Verification items for the finished model (mm, model axes). A direction names the side the tool comes from. Round coordinates to 2 decimals unless told otherwise and drop trailing zeros. Write each loop counter-clockwise with the first axis right and the second up, starting at its lowest first coordinate (ties: lowest second). Pieces come first, ordered by that corner, then holes. Notation, with made-up numbers: (44.5, 43) - (83.5, 43) arc R19 cw to (83.5, 57) - close; hole circle Ø7 at (64, 80). An arc over 180 degrees is marked (long way). Answer as a JSON object with one key per item and string values.
```python
from build123d import *

# Parameters (mm, degrees)
SKETCH_1_W              = 150
SKETCH_1_H              = 80
EXTRUDE_1_DEPTH         = 2
HOLE_WIZARD_3_2_3_2_1_D = 3.2
FILLET_1_R              = 5
SKETCH_4_W              = 25
SKETCH_4_H              = 60
CUT_EXTRUDE_1_DEPTH     = 86.023526156
FILLET_2_R              = 2


with BuildPart() as part:
    # 草图1 → 凸台-拉伸1 (new body)
    with BuildSketch(Plane(origin=(0, 0, 0), x_dir=(1, 0, 0), z_dir=(0, 1, 0))):
        Rectangle(SKETCH_1_W, SKETCH_1_H)
    extrude(amount=EXTRUDE_1_DEPTH)

    # Ø3.2 (3.2) 直径孔1 (through all)
    with Locations(Plane(origin=(-31, 2, -25), x_dir=(0, 0, 1), z_dir=(0, 1, 0))):
        with Locations((0, 0), (50, 0), (50, 62), (0, 62), (5, -39), (45, -39), (45, 101), (5, 101)):
            Hole(HOLE_WIZARD_3_2_3_2_1_D / 2)

    # 圆角1
    fillet_1_edges = [part.edges().sort_by_distance(p)[0] for p in [
        (75, 1, 40),
        (-75, 1, 40),
        (-75, 1, -40),
        (75, 1, -40),
    ]]
    fillet(fillet_1_edges, radius=FILLET_1_R)

    # 草图4 → 切除-拉伸1 (cut, through all)
    with BuildSketch(Plane(origin=(0, 2, 0), x_dir=(1, 0, 0), z_dir=(0, 1, 0))):
        with Locations((-47.5, 0)):
            Rectangle(SKETCH_4_W, SKETCH_4_H)
        Polygon((-27, 30), (-27, -20), (27, 30), align=None)
        Polygon((-23.081304406, -30), (27, -30), (27, 16.371578153), align=None)
        with Locations((47.5, 0)):
            Rectangle(SKETCH_4_W, SKETCH_4_H)
    extrude(amount=-CUT_EXTRUDE_1_DEPTH, mode=Mode.SUBTRACT)

    # 圆角2
    fillet_2_edges = [part.edges().sort_by_distance(p)[0] for p in [
        (-60, 1, 30),
        (-60, 1, -30),
        (-35, 1, -30),
        (-35, 1, 30),
        (-23.081304406, 1, 30),
        (27, 1, -16.371578153),
        (27, 1, 30),
        (-27, 1, -30),
        (27, 1, -30),
        (-27, 1, 20),
        (60, 1, -30),
        (60, 1, 30),
        (35, 1, 30),
        (35, 1, -30),
    ]]
    fillet(fillet_2_edges, radius=FILLET_2_R)


solid = part.part
```
Q1. Release check for a two-part mould opening along Z. For faces 1 (the flat face through (-1, 0, -1)), 2 (the cylindrical face through (73, 1, 39)), 3 (the cylindrical face through (-31.97, 0.99, 26.27)), 4 (the cylindrical face through (-74, 1, -38)) record: released by +Z, released by -Z, zero draft, split by the parting line, or undercut.
Geometry check:
{"face 1": "zero draft", "face 2": "released by +Z", "face 3": "undercut", "face 4": "released by -Z"}
Q2. Material ranges on line 1 along Z through (x, y) = (70, 1.6); line 2 along X through (y, z) = (1.65, -27); line 3 along Z through (x, y) = (46.5, 0.6), recorded low to high. Write a range as [from, to].
Geometry check:
{"line 1": "z = [-40, -21.6], [-18.4, 18.4], [21.6, 40]", "line 2": "x = [-75, -60], [-35, -27], [23.63, 35], [60, 75]", "line 3": "z = [-40, -30], [30, 40]"}
Q3. Set-up check for faces 5 (the flat face through (2.45, 1.01, 6.36)), 6 (the cylindrical face through (-74, 1, 38)): record each of +Z, -Z, +X, -X, +Y, -Y from which the full face is reachable in a straight line by a thin tool's end or side.
Geometry check:
{"face 5": "+Y, -Y", "face 6": "+Z, -X, +Y, -Y"}
Q4. Section check B-B, the plane z = -20. Record the cut outline in (x, y).
Geometry check:
{"outline": "(-75, 0) - (-71.6, 0) - (-71.6, 2) - (-75, 2) - close; (-68.4, 0) - (-60, 0) - (-60, 2) - (-68.4, 2) - close; (-35, 0) - (-27, 0) - (-27, 2) - (-35, 2) - close; (16.2, 0) - (35, 0) - (35, 2) - (16.2, 2) - close; (60, 0) - (68.4, 0) - (68.4, 2) - (60, 2) - close; (71.6, 0) - (75, 0) - (75, 2) - (71.6, 2) - close"}
Q5. Section check D-D, the plane x = 54. Record the cut outline in (y, z).
Geometry check:
{"outline": "(0, -40) - (2, -40) - (2, -30) - (0, -30) - close; (0, 30) - (2, 30) - (2, 40) - (0, 40) - close"}
Q6. Section check C-C, the plane z = -6. Record the cut outline in (x, y), then the cut area to 3 significant figures.
Geometry check:
{"outline": "(-75, 0) - (-60, 0) - (-60, 2) - (-75, 2) - close; (-35, 0) - (-27, 0) - (-27, 2) - (-35, 2) - close; (1.08, 0) - (15.8, 0) - (15.8, 2) - (1.08, 2) - close; (27, 0) - (35, 0) - (35, 2) - (27, 2) - close; (60, 0) - (75, 0) - (75, 2) - (60, 2) - close", "area": "121 mm2"}
Q7. Section check A-A, the plane x = 31. Record the cut outline in (y, z).
Geometry check:
{"outline": "(0, -40) - (2, -40) - (2, -26.6) - (0, -26.6) - close; (0, -23.4) - (2, -23.4) - (2, 23.4) - (0, 23.4) - close; (0, 26.6) - (2, 26.6) - (2, 40) - (0, 40) - close"}
